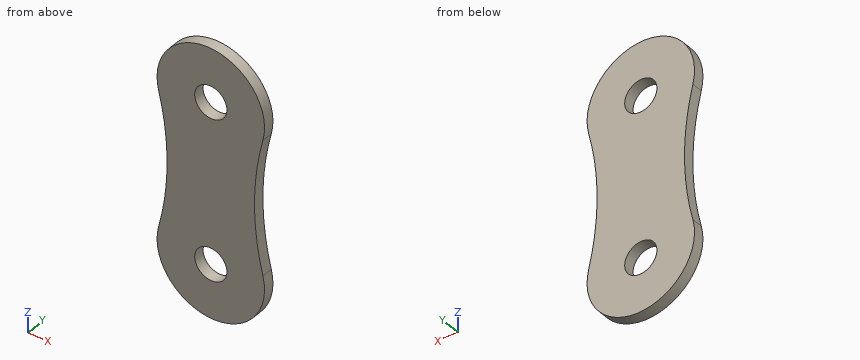
from build123d import *

# Parameters (mm, degrees)
F0_R     = 3.81
F1_DEPTH = 2.54


with BuildPart() as f1:
    # F0 (on Front) → F1 (new body)
    with BuildSketch(Plane.XZ):
        with BuildLine():
            ThreePointArc((12.312997, -15.938714), (10.330432, 0), (12.312997, 15.938714))
            ThreePointArc((12.312997, 15.938714), (0, 31.75), (-12.312997, 15.938714))
            ThreePointArc((-12.312997, 15.938714), (-10.330432, 0), (-12.312997, -15.938714))
            ThreePointArc((-12.312997, -15.938714), (0, -31.75), (12.312997, -15.938714))
        make_face()
        with Locations((0, -19.05)):
            Circle(F0_R, mode=Mode.SUBTRACT)
        with Locations((0, 19.05)):
            Circle(F0_R, mode=Mode.SUBTRACT)
    extrude(amount=F1_DEPTH)


solid = f1.part
Model file for the job. Use its own axes, mm. Give positions to 0.01 mm unless a question says otherwise; leave off trailing zeros. Write each loop counter-clockwise with the first axis right and the second up, starting at its lowest first coordinate (ties: lowest second). Pieces come first, ordered by that corner, then holes. Notation, with made-up numbers: (44, 15.25) -> (55, 15.25) arc R9 cw to (55, 26.25) -> close; hole circle Ø9 at (80.25, 74.25). An arc over 180 degrees is marked (long way). Write item = value, one per line.
(1) Slice it at C-C, the plane y = -1.1. Give the cut face in (x, z).
Determined:
outline = (-12.31, -15.94) arc R12.7 ccw (long way) to (12.31, -15.94) arc R65.06 cw to (12.31, 15.94) arc R12.7 ccw (long way) to (-12.31, 15.94) arc R65.06 cw to start; hole circle Ø7.62 at (0, -19.05); hole circle Ø7.62 at (0, 19.05)
(2) Slice it at D-D, the plane x = 2.75. Give the cut face in (y, z).
Determined:
outline = (-2.54, -31.45) -> (0, -31.45) -> (0, -21.69) -> (-2.54, -21.69) -> close; (-2.54, -16.41) -> (0, -16.41) -> (0, 16.41) -> (-2.54, 16.41) -> close; (-2.54, 21.69) -> (0, 21.69) -> (0, 31.45) -> (-2.54, 31.45) -> close
(3) Probe line 1 along Z through (x, y) = (-0.25, -2.2); line 2 along Z through (x, y) = (5.5, -0.5); line 3 along X through (y, z) = (-0.75, 27.5). List the from-to ranges inside material, lowest first.
Determined:
line_1 = -31.75 to -22.85, -15.25 to 15.25, 22.85 to 31.75
line_2 = -30.5 to 30.5
line_3 = -9.48 to 9.48
(4) Flat gauge pins, fed straight in: P1, Ø1, axis at x = 4, y = -2, coming from the -Z side; P2, Ø12, axis at x = 0, z = 19.05, coming from the -Y side; P3, Ø1.5, axis at y = -0.5, z = -7, coming from the -X side. Where does each tip first touch, or does it go through?
Determined:
P1 = -31.26
P2 = -2.54
P3 = -10.79
(5) Slice it at A-A, the plane z = -19.05. Give the cut face in (x, y).
Determined:
outline = (-12.7, -2.54) -> (-3.81, -2.54) -> (-3.81, 0) -> (-12.7, 0) -> close; (3.81, -2.54) -> (12.7, -2.54) -> (12.7, 0) -> (3.81, 0) -> close
(6) Slice it at B-B, the plane x = 0. Give the cut face in (y, z), then the cut area to 3 significant figures.
Determined:
outline = (-2.54, -31.75) -> (0, -31.75) -> (0, -22.86) -> (-2.54, -22.86) -> close; (-2.54, -15.24) -> (0, -15.24) -> (0, 15.24) -> (-2.54, 15.24) -> close; (-2.54, 22.86) -> (0, 22.86) -> (0, 31.75) -> (-2.54, 31.75) -> close
area = 123 mm2
